The listing builds one solid part. Answer for the finished solid, in the listing's coordinates (mm). A direction names the side the tool comes from. Give positions to 0.01 mm unless a question says otherwise; leave off trailing zeros. Order: outer loops, then holes, each group sorted by start corner. A loop starts at its lowest first (then second) coordinate and runs counter-clockwise, first axis right, second up. Notation, with made-up numbers: M 61,51.25 L 109,51.25 A33 cw 109,89.25 Z; hole C 18,30.5 d9. An arc over 180 degrees is marked long. Answer as a JSON object with one key per item and string values. Group by question number.
```python
from build123d import *

# Parameters (mm, degrees)
SKETCH1_W           = 60
SKETCH1_H           = 50
BOSS_EXTRUDE1_DEPTH = 5.08
SKETCH2_OUTSIDE_W   = 77.654
SKETCH2_OUTSIDE_H   = 67.654
SKETCH2_OUTSIDE_R   = 3.675
CUT_EXTRUDE1_DEPTH  = 56.468381585
SKETCH12_W          = 20
SKETCH12_H          = 3
CUT_EXTRUDE6_DEPTH  = 10
SKETCH13_W          = 20
SKETCH13_H          = 3
CUT_EXTRUDE7_DEPTH  = 10
SKETCH14_W          = 40
SKETCH14_H          = 20
CUT_EXTRUDE8_DEPTH  = 2
SKETCH15_R          = 2
CUT_EXTRUDE9_DEPTH  = 56.468381585


with BuildPart() as part:
    # Sketch1 → Boss-Extrude1 (new body)
    with BuildSketch(Plane(origin=(0, 0, 0), x_dir=(1, 0, 0), z_dir=(0, 1, 0))):
        with Locations((-18.058684047, 2.226785401)):
            Rectangle(SKETCH1_W, SKETCH1_H)
    extrude(amount=BOSS_EXTRUDE1_DEPTH)

    # Sketch2 outside → Cut-Extrude1 (cut, through all)
    # profile 1 of 3: a face of its own
    with BuildSketch(Plane(origin=(0, 5.08, 0), x_dir=(1, 0, 0), z_dir=(0, 1, 0))):
        with Locations((-18.059, 2.227)):
            Rectangle(SKETCH2_OUTSIDE_W, SKETCH2_OUTSIDE_H)
        Polygon((-30.758684047, 27.226785401), (-5.358684047, 27.226785401), (11.941315953, 15.226785401), (11.941315953, -10.773214599), (-5.358684047, -22.773214599), (-30.758684047, -22.773214599), (-48.058684047, -10.773214599), (-48.058684047, 15.226785401), align=None, mode=Mode.SUBTRACT)
    # profile 2 of 3: a face of its own
    with BuildSketch(Plane(origin=(0, 5.08, 0), x_dir=(1, 0, 0), z_dir=(0, 1, 0))):
        with Locations(Location((-18.058684047, 19.726785401, 0), (0, 0, 270))):
            Circle(SKETCH2_OUTSIDE_R)
    # profile 3 of 3: a face of its own
    with BuildSketch(Plane(origin=(0, 5.08, 0), x_dir=(1, 0, 0), z_dir=(0, 1, 0))):
        with Locations(Location((-18.058684047, -15.273214599, 0), (0, 0, 90))):
            Circle(SKETCH2_OUTSIDE_R)
    extrude(amount=-CUT_EXTRUDE1_DEPTH, mode=Mode.SUBTRACT)

    # Sketch12 → Cut-Extrude6 (cut)
    with BuildSketch(Plane.ZY.offset(48.058684047)):
        with Locations((-2.185006669, 1.5)):
            Rectangle(SKETCH12_W, SKETCH12_H)
    extrude(amount=-CUT_EXTRUDE6_DEPTH, mode=Mode.SUBTRACT)

    # Sketch13 → Cut-Extrude7 (cut)
    with BuildSketch(Plane(origin=(11.941315953, 0, 0), x_dir=(0, 0, -1), z_dir=(1, 0, 0))):
        with Locations((2.226785401, 1.5)):
            Rectangle(SKETCH13_W, SKETCH13_H)
    extrude(amount=-CUT_EXTRUDE7_DEPTH, mode=Mode.SUBTRACT)

    # Sketch14 → Cut-Extrude8 (cut)
    with BuildSketch(Plane(origin=(0, 5.08, 0), x_dir=(1, 0, 0), z_dir=(0, 1, 0))):
        with Locations((-18.058684047, 2.226785401)):
            Rectangle(SKETCH14_W, SKETCH14_H)
    extrude(amount=-CUT_EXTRUDE8_DEPTH, mode=Mode.SUBTRACT)

    # Sketch15 → Cut-Extrude9 (cut, through all)
    with BuildSketch(Plane(origin=(0, 5.08, 0), x_dir=(1, 0, 0), z_dir=(0, 1, 0))):
        with Locations(Location((-43.015186805, -2.773214599, 0), (0, 0, 270))):
            Circle(SKETCH15_R)
        with Locations(Location((-43.081568636, 7.292867381, 0), (0, 0, 270))):
            Circle(SKETCH15_R)
        with Locations(Location((6.964200542, 7.292867381, 0), (0, 0, 270))):
            Circle(SKETCH15_R)
        with Locations(Location((6.89781871, -2.773214599, 0), (0, 0, 270))):
            Circle(SKETCH15_R)
    extrude(amount=-CUT_EXTRUDE9_DEPTH, mode=Mode.SUBTRACT)


solid = part.part
```
Item 1: Section D-D (y = 0.7) is taken. Determine the outline of the cut face in (x, z) (3 decimals), and give its area (3 significant figures).
Item 2: Section C-C (x = -19) is taken. Determine the outline of the cut face in (y, z), and give its area (3 significant figures).
Item 3: Consider probe 1 along X at (y, z) = (3.55, 3); probe 2 along X at (y, z) = (4.6, -5); probe 3 along Z at (x, y) = (8, 4). Determine where each line is inside the solid, lowest interval first. Write a range as from..to.
Item 4: Flat-ended cylindrical pins translate along their axes: P1, Ø1.5, axis at x = 5.5, y = 1, coming from the -Z side (3 decimals); P2, Ø5, axis at x = -43.02, z = 2.77, coming from the -Y side; P3, Ø1.5, axis at x = 6, y = 1.5, coming from the +Z side; P4, Ø10, axis at x = 1.5, z = 9.5, coming from the -Y side. Find the tip coordinate at first contact, or state that the pin passes through.
Item 5: Section A-A (z = 13) is taken. Determine the outline of the cut face in (x, y).
Item 6: A tool of negligible diameter and unlimited length cuts with its end or side. For faces 1 (the flat face through (-38.059, 4, -2)), 2 (the flat face through (-39.288, 2.576, 16.857)), 3 (the flat face through (-43, 1, -12.185)), from which of +Z, -Z, +X, -X, +Y, -Y can it reach the whole face along a straight path? Write none if from no direction.
Item 7: Determine the mould class of faces 4 (the flat face through (-39.53, 2.576, -21.143)), 5 (the cylindrical face through (-44.79, 4.055, 3.696)), 6 (the flat face through (1.941, 2, -2)), 7 (the flat face through (7, 3, -2)) for opening direction X: released by +X, released by -X, zero draft, split by the parting line, or undercut.
Item 8: Section B-B (y = 4.3) is taken. Determine the outline of the cut face in (x, z) (3 decimals).
Values found:
{
 "1": {"outline": "M -48.059,-15.227 L -30.759,-27.227 L -5.359,-27.227 L 11.941,-15.227 L 11.941,-12.227 L 1.941,-12.227 L 1.941,7.773 L 11.941,7.773 L 11.941,10.773 L -5.359,22.773 L -30.759,22.773 L -48.059,10.773 L -48.059,7.815 L -38.059,7.815 L -38.059,-12.185 L -48.059,-12.185 Z; hole C -18.059,-19.727 d7.35; hole C -18.059,15.273 d7.35", "area": "2,100 mm^2"},
 "2": {"outline": "M 0,-27.23 L 5.08,-27.23 L 5.08,-23.28 L 0,-23.28 Z; M 0,-16.17 L 5.08,-16.17 L 5.08,-12.23 L 3.08,-12.23 L 3.08,7.77 L 5.08,7.77 L 5.08,11.72 L 0,11.72 Z; M 0,18.83 L 5.08,18.83 L 5.08,22.77 L 0,22.77 Z", "area": "142 mm^2"},
 "3": {"probe 1": "x = -48.06..-45, -41.03..-38.06, 1.94..4.91, 8.88..11.94", "probe 2": "x = -48.06..-38.06, 1.94..11.94", "probe 3": "z = -17.96..-9, -5.58..1.1, 4.44..13.51"},
 "4": {"P1": "stops at z = -20.215", "P2": "stops at y = 3", "P3": "stops at z = 15.41", "P4": "stops at y = 0"},
 "5": {"outline": "M -44.85,0 L -20.95,0 L -20.95,5.08 L -44.85,5.08 Z; M -15.17,0 L 8.73,0 L 8.73,5.08 L -15.17,5.08 Z"},
 "6": {"face 1": "+Y", "face 2": "+Z, -X, +Y, -Y", "face 3": "-X, -Y"},
 "7": {"face 4": "released by -X", "face 5": "undercut", "face 6": "released by +X", "face 7": "zero draft"},
 "8": {"outline": "M -48.059,-15.227 L -30.759,-27.227 L -5.359,-27.227 L 11.941,-15.227 L 11.941,10.773 L -5.359,22.773 L -30.759,22.773 L -48.059,10.773 Z; hole C -43.082,-7.293 d4; hole C -43.015,2.773 d4; hole M -38.059,-12.227 L 1.941,-12.227 L 1.941,7.773 L -38.059,7.773 Z; hole C -18.059,-19.727 d7.35; hole C -18.059,15.273 d7.35; hole C 6.898,2.773 d4; hole C 6.964,-7.293 d4"}
}
